Autodesk Inventor part; units mm, degrees
ref_plane "YZ Plane" through (0, 0, 0) normal (1, 0, 0) x (0, 1, 0)
ref_plane "XZ Plane" through (0, 0, 0) normal (0, 1, 0) x (-1, 0, 0)
ref_plane "XY Plane" through (0, 0, 0) normal (0, 0, 1) x (1, 0, 0)
sketch "Sketch1" plane through (0, 0, 0) normal (0, 1, 0) x (-1, 0, 0)
  circle A0 centre (0, 0) radius 4.5
  dimension "d0" = 9
extrude "Extrusion1" add sketch "Sketch1" along normal blind 0.5
sketch "Sketch2" plane through (0, 0, 0) normal (0, -1, 0) x (1, 0, 0)
  circle A0 centre (0, 0) radius 2.5
  dimension "d3" = 5
extrude "Extrusion2" add sketch "Sketch2" along normal blind 20
chamfer "Chamfer1" distance 2.5 angle 45 1 edges at (-2.5, -20, 0)
properties part number "Pin"
Read the model definition and answer for the solid it produces. Units are mm, in the model's axes. A direction names the side the tool comes from. Round coordinates to 2 decimals unless told otherwise and drop trailing zeros. Order: outer loops, then holes, each group sorted by start corner. A loop starts at its lowest first (then second) coordinate and runs counter-clockwise, first axis right, second up.
1) Straight lines are drawn through the part: L1, parallel to Y at x = -3.5, z = -2; L2, parallel to Z at x = 0, y = -14.25; L3, parallel to X at y = -5.25, z = -1.5. For each, find the intervals that lie inside material, in ascending order.
2) The part is cut by section A-A on y = -3. Write down the section's boundary in (x, z).
3) The part is cut by section B-B on x = -3. Write down the section's boundary in (y, z), plus the area to 3 significant figures.
4) For faces 1 (the face through (-0.54, -8.63, 2.44)), 2 (the face through (0, 0.5, 0)), determine the directions among +Z, -Z, +X, -X, +Y, -Y from which every point of the face is accessible in a straight line to the end or side of a thin tool.
5) Flat-ended cylindrical pins translate along their axes: pin 1 (1.5 mm diameter, centred on x = 1, y = -9, fed in from -Z); pin 2 (3 mm diameter, centred on x = 3, y = -4.5, fed in from +Z); pin 3 (1 mm diameter, centred on y = -6.5, z = 0.5, fed in from -X). Find the tip coordinate at first contact, or state that the pin passes through.
6) The part is cut by section C-C on z = -3.5. Write down the section's boundary in (x, y), plus the area to 3 significant figures.
Resolved:
1. L1: y = 0 to 0.5
1. L2: z = -2.5 to 2.5
1. L3: x = -2 to 2
2. outline: circle Ø5 at (0, 0)
3. outline: (0, -3.35) - (0.5, -3.35) - (0.5, 3.35) - (0, 3.35) - close
3. area: 3.35 mm2
4. face 1: -Y
4. face 2: +Z, -Z, +X, -X, +Y
5. pin 1: stops at z = -2.49
5. pin 2: stops at z = 2
5. pin 3: stops at x = -2.5
6. outline: (-2.83, 0) - (2.83, 0) - (2.83, 0.5) - (-2.83, 0.5) - close
6. area: 2.83 mm2
